The figure shows three views and two pictorial views of one solid part (mm, origin at its lowest corner). Answer the questions. A direction names the side the tool comes from. Give positions to 0.01 mm unless a question says otherwise; leave off trailing zeros. Loops run counter-clockwise (first coordinate to the right, second up) from the corner with the lowest first, then second, coordinate; pieces in that order, holes last. Notation, with made-up numbers: M -9.5,62 L 11.5,62 A13 ccw 11.5,74 Z; hole C 51.25,47.25 d6. An arc over 180 degrees is marked long. One line per item, written item: value. Start each with the question number.
Q1. A cutting plane is placed at A-A, the plane y = 16.5. State how many separate pieces and enclosed holes the cut face has, and give its area (3 significant figures).
Q2. A cutting plane is placed at B-B, the plane z = 101. Determine the outline of the cut face in (x, y), and give its area (3 significant figures).
Q3. Consider L1, parallel to X at y = 22.5, z = 455; L2, parallel to Z at x = 200, y = 19.5; L3, parallel to X at y = 12.25, z = 451. Determine where each line is inside the solid, lowest interval first.
Q4. The mould has two halves that part along Z. Classify the marked faces 3, 4 and 5: +Z half, -Z half, draft (parallel to the pull), parting line (faces both ways), or undercut.
Q5. A cutting plane is placed at C-C, the plane x = 200. Determine the outline of the cut face in (y, z), and give its area (3 significant figures).
Q6. A flat-ended cylindrical pin translates along its axis: pin 1 (6 mm diameter, centred on x = 319, y = 26, fed in from -Z). Find the tip coordinate at first contact, or state that the pin passes through.
Q7. A cutting plane is placed at D-D, the plane z = 325. Determine the outline of the cut face in (x, y), and give its area (3 significant figures).
Q8. For the marked faces 1 and 2, determine the directions among +Z, -Z, +X, -X, +Y, -Y from which every point of the face is accessible in a straight line to the end or side of a thin tool.
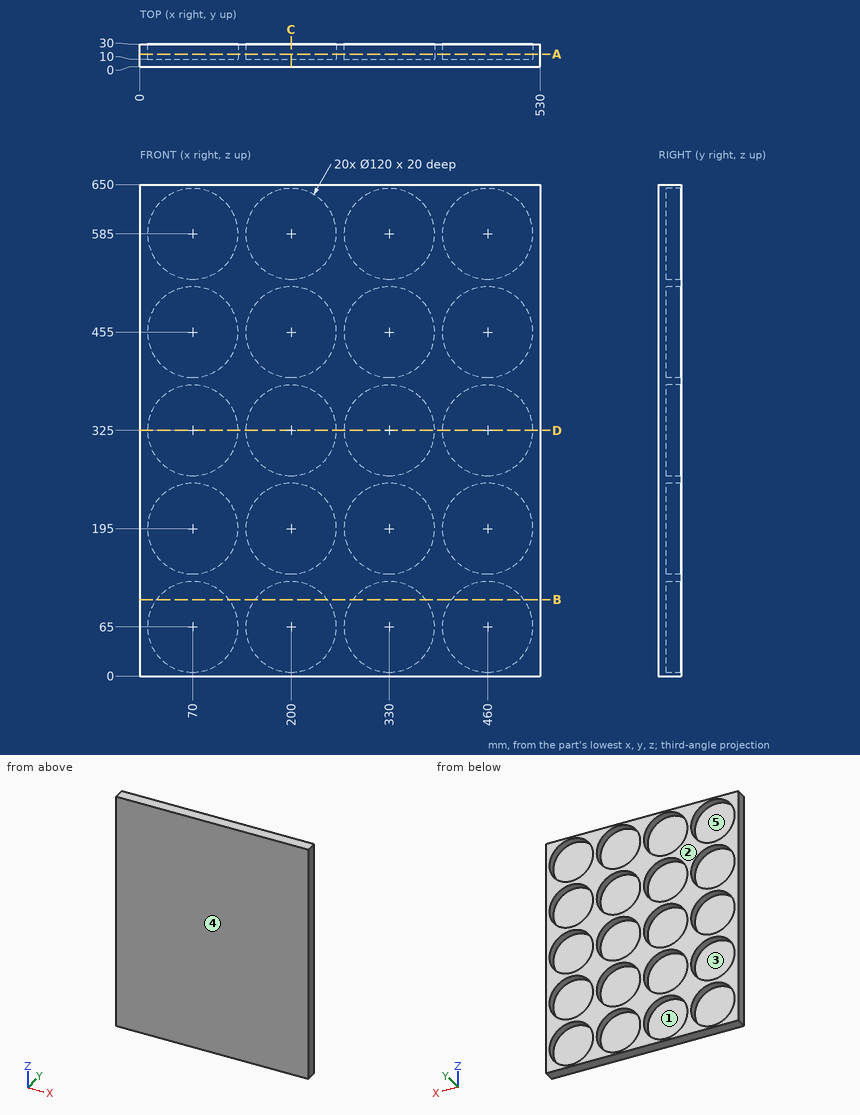
Answer block:
1. separate pieces: 1
1. enclosed holes: 20
1. area: 118,000 mm^2
2. outline: M 0,0 L 530,0 L 530,30 L 508,30 L 508,10 L 412,10 L 412,30 L 378,30 L 378,10 L 282,10 L 282,30 L 248,30 L 248,10 L 152,10 L 152,30 L 118,30 L 118,10 L 22,10 L 22,30 L 0,30 Z
2. area: 8,220 mm^2
3. L1: 0 to 10, 130 to 140, 260 to 270, 390 to 400, 520 to 530
3. L2: 0 to 5, 125 to 135, 255 to 265, 385 to 395, 515 to 525, 645 to 650
3. L3: 0 to 10.13, 129.87 to 140.13, 259.87 to 270.13, 389.87 to 400.13, 519.87 to 530
4. face 3: undercut
4. face 4: draft
4. face 5: undercut
5. outline: M 0,0 L 30,0 L 30,5 L 10,5 L 10,125 L 30,125 L 30,135 L 10,135 L 10,255 L 30,255 L 30,265 L 10,265 L 10,385 L 30,385 L 30,395 L 10,395 L 10,515 L 30,515 L 30,525 L 10,525 L 10,645 L 30,645 L 30,650 L 0,650 Z
5. area: 7,500 mm^2
6. pin 1: z = 0
7. outline: M 0,0 L 530,0 L 530,30 L 520,30 L 520,10 L 400,10 L 400,30 L 390,30 L 390,10 L 270,10 L 270,30 L 260,30 L 260,10 L 140,10 L 140,30 L 130,30 L 130,10 L 10,10 L 10,30 L 0,30 Z
7. area: 6,300 mm^2
8. face 1: +Y
8. face 2: +Z, -Z, +X, -X, +Y
